Geometry: final body of the model. Coordinates: model frame, mm. Face numbers are marked on the shaded views. A direction names the side the tool comes from. Coordinates: 2 decimals unless noted, no trailing zeros. Write each loop counter-clockwise with the first axis right and the second up, starting at its lowest first coordinate (ties: lowest second). Pieces come first, ordered by that corner, then holes. Notation, with made-up numbers: (50, -11.75) - (102, -11.75) arc R28 ccw to (102, 23.25) - close; hole circle Ø6 at (5, 46.5). An arc over 180 degrees is marked (long way). Answer as a JSON object with one key per item and string values. Group by question number.
Item 1: First-contact query: pin 1 Ø8 at (y, z) = (2.5, 6) entering from -X; pin 2 Ø3 at (x, y) = (-9, 19) entering from -Z; pin 3 Ø1 at (x, y) = (-10.5, 17) entering from +Z. Flat tips, straight axial feed; report the tip coordinate or a pass-through.
Item 2: Set-up query: the marked faces 4, 5, 6, 7 and 8. Return all of +Z, -Z, +X, -X, +Y, -Y with unobstructed straight access to the full face (end or side cutting, diameter ignored); none if empty.
Item 3: Section A-A on z = 0. Return loops of the section in (x, y).
Item 4: Section B-B on x = 0. Return loops of the section in (y, z).
Item 5: Line query: line 1 along X through (y, z) = (-0.45, 0); line 2 along X through (y, z) = (-5.75, 0); line 3 along X through (y, z) = (23.5, 9). Output: solid intervals per line, ascending. Write a range as from..to.
Item 6: Section D-D on x = -3.5. Return loops of the section in (y, z).
Item 7: Mould query, pull axis Z, two halves, no side actions, for the marked faces 1, 2 and 3. Classes: pulls with the +Z half, pulls with the -Z half, needs draft (parallel to the pull), parting line crosses it, or undercut.
Item 8: Section C-C on y = 14. Return loops of the section in (x, z), and give its area (3 significant figures).
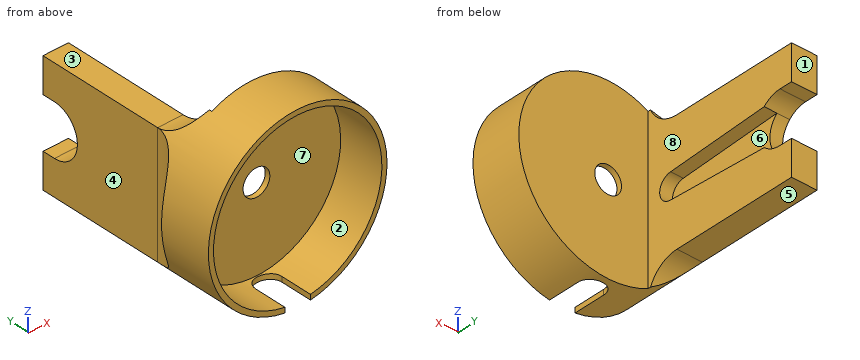
```python
from build123d import *

# Parameters (mm, degrees)
SKETCH1_R           = 14
BOSS_EXTRUDE1_DEPTH = 8
SHELL1_T            = -0.8
SKETCH2_R           = 2.1
CUT_EXTRUDE1_DEPTH  = 2
SKETCH3_W           = 4
SKETCH3_H           = 19
BOSS_EXTRUDE2_DEPTH = 25
CUT_EXTRUDE2_DEPTH  = 19
SKETCH4_3_R         = 2
CUT_EXTRUDE3_DEPTH  = 2
FILLET1_R           = 5
FILLET2_R           = 5
CUT_EXTRUDE4_DEPTH  = 20


with BuildPart() as part:
    # Sketch1 → Boss-Extrude1 (new body)
    with BuildSketch(Plane(origin=(0, 0, 0), x_dir=(1, 0, 0), z_dir=(0, 1, 0))):
        with Locations(Location((0, 0, 0), (0, 0, 270))):
            Circle(SKETCH1_R)
    extrude(amount=-BOSS_EXTRUDE1_DEPTH)

    # Shell1
    shell1_openings = [part.faces().sort_by_distance(p)[0] for p in [
        (0, -8, 0),
    ]]
    offset(amount=SHELL1_T, openings=shell1_openings, kind=Kind.INTERSECTION)

    # Sketch2 → Cut-Extrude1 (cut)
    with BuildSketch(Plane(origin=(0, 0, 0), x_dir=(1, 0, 0), z_dir=(0, 1, 0))):
        with Locations(Location((0, 0, 0), (0, 0, 270))):
            Circle(SKETCH2_R)
    extrude(amount=-CUT_EXTRUDE1_DEPTH, mode=Mode.SUBTRACT)

    # Sketch3 → Boss-Extrude2 (add)
    with BuildSketch(Plane(origin=(0, 0, 0), x_dir=(1, 0, 0), z_dir=(0, 1, 0))):
        with Locations((-8.283481901, 0)):
            Rectangle(SKETCH3_W, SKETCH3_H)
    extrude(amount=BOSS_EXTRUDE2_DEPTH)

    # Sketch4 → Cut-Extrude2 (cut)
    with BuildSketch(Plane(origin=(-6.283481901, 0, 0), x_dir=(0, 0, -1), z_dir=(1, 0, 0))):
        with BuildLine():
            ThreePointArc((-4, 23), (-3.712354677, 21.510562941), (-2.890788624, 20.235340684))
            ThreePointArc((-2.890788624, 20.235340684), (0, 19), (2.890788624, 20.235340684))
            ThreePointArc((2.890788624, 20.235340684), (3.712354677, 21.510562941), (4, 23))
            Line((4, 23), (4, 25))
            Line((4, 25), (-4, 25))
            Line((-4, 25), (-4, 23))
        make_face()
    extrude(amount=-CUT_EXTRUDE2_DEPTH, mode=Mode.SUBTRACT)

    # Sketch4<3> → Cut-Extrude3 (cut)
    with BuildSketch(Plane(origin=(-6.283481901, 0, 0), x_dir=(0, 0, -1), z_dir=(1, 0, 0))):
        with BuildLine():
            ThreePointArc((2.890788624, 20.235340684), (0, 19), (-2.890788624, 20.235340684))
            Line((-2.890788624, 20.235340684), (-1.997016436, 3.890796724))
            ThreePointArc((-1.997016436, 3.890796724), (-0.054622013, 5.99925397), (2, 4))
            ThreePointArc((2, 4), (1.99925397, 3.945377987), (1.997016436, 3.890796724))
            Line((1.997016436, 3.890796724), (2.890788624, 20.235340684))
        make_face()
        with Locations((0, 4)):
            Circle(SKETCH4_3_R)
    extrude(amount=-CUT_EXTRUDE3_DEPTH, mode=Mode.SUBTRACT)

    # Fillet1
    # the kernel refuses this fillet: 5 mm, written as the material it adds along each edge
    with BuildSketch(Plane(origin=(-10.283481901, 0, 9.5), x_dir=(-1, 0, 0), z_dir=(0, 0, -1))) as fillet1_piece_1_section:
        with BuildLine():
            CenterArc((FILLET1_R, FILLET1_R), FILLET1_R, 180, 90)
            Line((0, FILLET1_R), (0, 0))
            Line((0, 0), (FILLET1_R, 0))
        make_face()
    fillet1_piece_1 = extrude(amount=19, mode=Mode.PRIVATE)
    fillet1_piece_1 = fillet1_piece_1 & Plane(origin=(0, 1.284116868, 0), x_dir=(0, 0, 1), z_dir=(0, 1, 0)) * Cylinder(14, 58, mode=Mode.PRIVATE)
    add(fillet1_piece_1)

    # Fillet2
    # the kernel refuses this fillet: 5 mm, written as the material it adds along each edge
    with BuildSketch(Plane(origin=(-22.783481901, 0, -9.5), x_dir=(0, 1, 0), z_dir=(1, 0, 0))) as fillet2_piece_1_section:
        with BuildLine():
            CenterArc((FILLET2_R, -FILLET2_R), FILLET2_R, 90, 90)
            Line((0, -FILLET2_R), (0, 0))
            Line((0, 0), (FILLET2_R, 0))
        make_face()
    fillet2_piece_1 = extrude(amount=16.5, mode=Mode.PRIVATE)
    fillet2_piece_1 = fillet2_piece_1 & Plane(origin=(0, 1.41467333, 0), x_dir=(0, 0, 1), z_dir=(0, 1, 0)) * Cylinder(14, 53, mode=Mode.PRIVATE)
    add(fillet2_piece_1)
    with BuildSketch(Plane(origin=(-6.283481901, 0, 9.5), x_dir=(0, 1, 0), z_dir=(-1, 0, 0))) as fillet2_piece_2_section:
        with BuildLine():
            CenterArc((FILLET2_R, -FILLET2_R), FILLET2_R, 90, 90)
            Line((0, -FILLET2_R), (0, 0))
            Line((0, 0), (FILLET2_R, 0))
        make_face()
    fillet2_piece_2 = extrude(amount=16.5, mode=Mode.PRIVATE)
    fillet2_piece_2 = fillet2_piece_2 & Plane(origin=(0, 1.414673355, 0), x_dir=(0, 0, 1), z_dir=(0, 1, 0)) * Cylinder(14, 53, mode=Mode.PRIVATE)
    add(fillet2_piece_2)

    # Sketch5 → Cut-Extrude4 (cut)
    with BuildSketch(Plane.XY):
        with BuildLine():
            Line((-2, -3), (-2, -8))
            Line((-2, -8), (2, -8))
            Line((2, -8), (2, -3))
            ThreePointArc((2, -3), (0, -1), (-2, -3))
        make_face()
    extrude(amount=-CUT_EXTRUDE4_DEPTH, mode=Mode.SUBTRACT)


solid = part.part
```
Checks:
{
 "1": {"pin 1": "x = -13.74", "pin 2": "z = -9.5", "pin 3": "z = 9.5"},
 "2": {"face 4": "+Z, -Z, -X, +Y", "face 5": "-Z, +X, -X, +Y", "face 6": "+X, +Y", "face 7": "-Y", "face 8": "+Z, -Z, +X, +Y"},
 "3": {"outline": "(-14, -8) - (-13.2, -8) - (-13.2, -0.8) - (-2.1, -0.8) - (-2.1, 0) - (-6.28, 0) - (-6.28, 2) - (-8.28, 2) - (-8.28, 19) - (-10.28, 19) - (-10.28, 5) arc R5 cw to (-14, 0.17) - close; (2.1, -0.8) - (13.2, -0.8) - (13.2, -8) - (14, -8) - (14, 0) - (2.1, 0) - close"},
 "4": {"outline": "(-8, 13.2) - (-0.8, 13.2) - (-0.8, 2.1) - (0, 2.1) - (0, 14) - (-8, 14) - close; (-1, -14) - (0, -14) - (0, -2.1) - (-0.8, -2.1) - (-0.8, -13.2) - (-1, -13.2) - close"},
 "5": {"line 1": "-14..-2.1, 2.1..14", "line 2": "-14..-13.2, 13.2..14", "line 3": "-10.28..-6.28"},
 "6": {"outline": "(-8, -13.56) - (0, -13.56) - (0, 13.56) - (-8, 13.56) - (-8, 12.73) - (-0.8, 12.73) - (-0.8, -12.73) - (-8, -12.73) - close"},
 "7": {"face 1": "needs draft", "face 2": "undercut", "face 3": "pulls with the +Z half"},
 "8": {"outline": "(-10.28, -9.5) - (-6.28, -9.5) - (-6.28, -2.55) - (-8.28, -2.55) - (-8.28, 2.55) - (-6.28, 2.55) - (-6.28, 9.5) - (-10.28, 9.5) - close", "area": "65.8 mm^2"}
}
